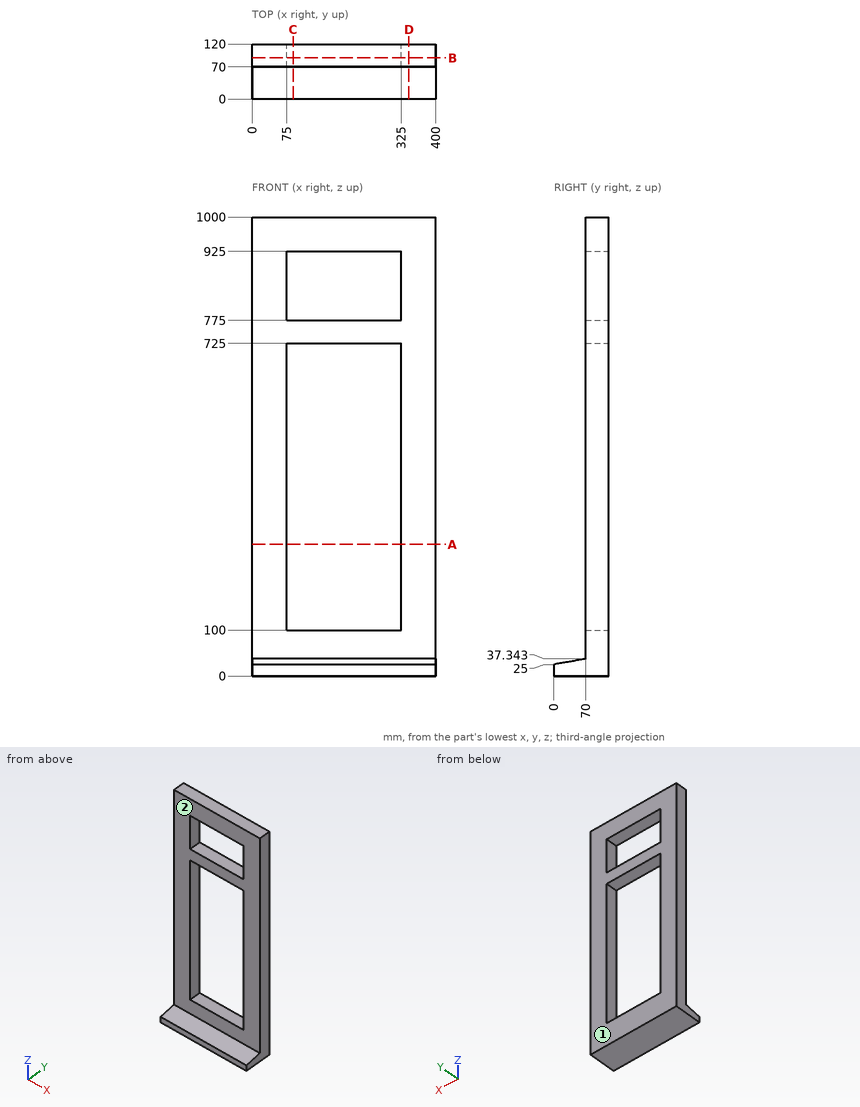
Geometry: see drawing. Coordinates: mm, zero at the bounding-box minimum. A direction names the side the tool comes from. Give positions to 0.01 mm unless a question says otherwise; leave off trailing zeros. Loops run counter-clockwise (first coordinate to the right, second up) from the corner with the lowest first, then second, coordinate; pieces in that order, holes last. Notation, with made-up numbers: (61.25, -33.5) - (120.25, -33.5) arc R11 ccw to (120.25, -17.5) - close; hole circle Ø4 at (85, 58). An arc over 180 degrees is marked (long way). One line per question, with ' | ' between items. Start each with the question number.
(1) Reachability of the marked faces 1 and 2 from +Z, -Z, +X, -X, +Y, -Y: full face, straight path, thin tool, end or side. Return the list, or none.
(2) Contact query for a flat-ended pin moving along its axis: pin 1 (3 mm diameter, centred on x = 50, z = 862.5, fed in from -Y). Output: stop coordinate, or through.
(3) Ray query, line 1 (Z direction, x = 94, y = 111); line 2 (X direction, y = 79, z = 788); line 3 (Y direction, x = 380.5, z = 886). Return the intervals inside material, ascending. Write a range as from..to.
(4) Section query A-A on z = 287. Return loops of the section in (x, y), then the cut area to 3 significant figures.
(5) Section query D-D on x = 341.5. Return loops of the section in (y, z), then the cut area to 3 significant figures.
(6) Section query C-C on x = 89. Return loops of the section in (y, z), then the cut area to 3 significant figures.
(7) Section query B-B on y = 90. Return loops of the section in (x, z), then the cut area to 3 significant figures.
The answers:
1) face 1: +Z, -Z, +X, -X, +Y | face 2: +Z, +X, -X, -Y
2) pin 1: y = 70
3) line 1: 0..100, 725..775, 925..1000 | line 2: 0..75, 325..400 | line 3: 70..120
4) outline: (0, 70) - (75, 70) - (75, 120) - (0, 120) - close; (325, 70) - (400, 70) - (400, 120) - (325, 120) - close | area: 7,500 mm2
5) outline: (0, 0) - (120, 0) - (120, 1000) - (70, 1000) - (70, 37.34) - (0, 25) - close | area: 52,200 mm2
6) outline: (0, 0) - (120, 0) - (120, 100) - (70, 100) - (70, 37.34) - (0, 25) - close; (70, 725) - (120, 725) - (120, 775) - (70, 775) - close; (70, 925) - (120, 925) - (120, 1000) - (70, 1000) - close | area: 13,400 mm2
7) outline: (0, 0) - (400, 0) - (400, 1000) - (0, 1000) - close; hole (75, 100) - (325, 100) - (325, 725) - (75, 725) - close; hole (75, 775) - (325, 775) - (325, 925) - (75, 925) - close | area: 206,000 mm2
